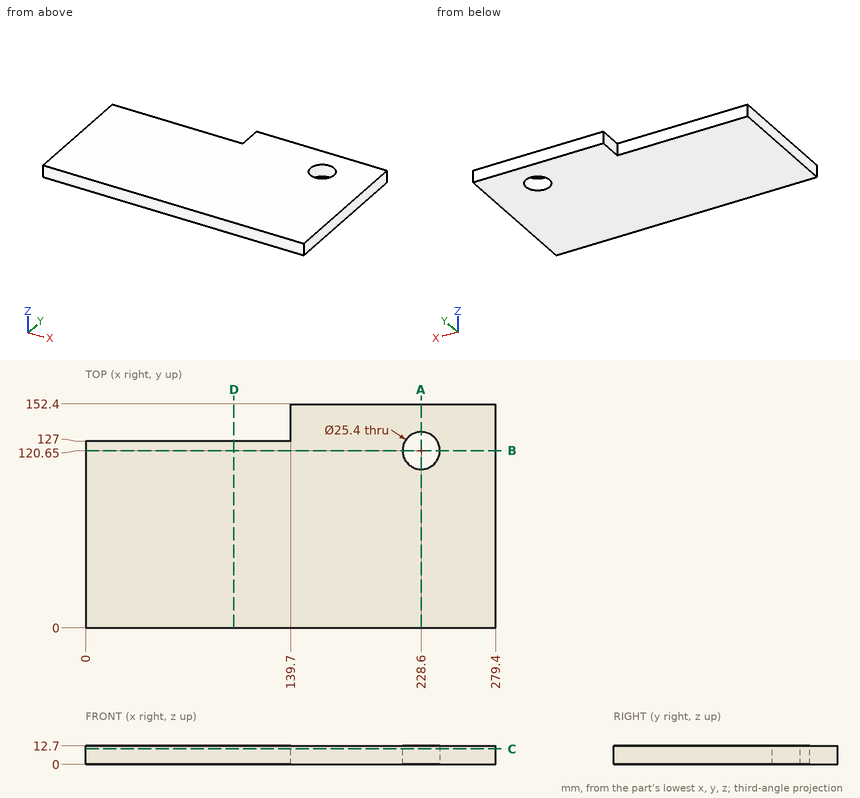
Here's the drawing with two shaded views (mm, measured from the low corner). I have some questions. Round coordinates to 2 decimals unless told otherwise and drop trailing zeros. Loops run counter-clockwise (first coordinate to the right, second up) from the corner with the lowest first, then second, coordinate; pieces in that order, holes last.
Item 1: Suppose I cut it at D-D, the plane x = 101. Write out the boundary of the cut face in (y, z), then the cut area to 3 significant figures.
Item 2: Will this pin go through, and if not, where does the flat tip stop? pin 1 Ø1 at (x, y) = (136.5, 79.5) entering from -Z.
Item 3: Suppose I cut it at A-A, the plane x = 228.6. Write out the boundary of the cut face in (y, z), then the cut area to 3 significant figures.
Item 4: Please list where these lines run through material, in increasing order: L1, parallel to Y at x = 228.6, z = 3; L2, parallel to Y at x = 109, z = 6.5; L3, parallel to X at y = 119, z = 2.75.
Item 5: Suppose I cut it at C-C, the plane z = 10.5. Write out the boundary of the cut face in (x, y).
Item 6: Suppose I cut it at B-B, the plane y = 120.65. Write out the boundary of the cut face in (x, z), then the cut area to 3 significant figures.
Reported:
1. outline: (0, 0) - (127, 0) - (127, 12.7) - (0, 12.7) - close
1. area: 1,610 mm2
2. pin 1: stops at z = 0
3. outline: (0, 0) - (107.95, 0) - (107.95, 12.7) - (0, 12.7) - close; (133.35, 0) - (152.4, 0) - (152.4, 12.7) - (133.35, 12.7) - close
3. area: 1,610 mm2
4. L1: y = 0 to 107.95, 133.35 to 152.4
4. L2: y = 0 to 127
4. L3: x = 0 to 216.01, 241.19 to 279.4
5. outline: (0, 0) - (279.4, 0) - (279.4, 152.4) - (139.7, 152.4) - (139.7, 127) - (0, 127) - close; hole circle Ø25.4 at (228.6, 120.65)
6. outline: (0, 0) - (215.9, 0) - (215.9, 12.7) - (0, 12.7) - close; (241.3, 0) - (279.4, 0) - (279.4, 12.7) - (241.3, 12.7) - close
6. area: 3,230 mm2
